Part model, mm, in its own coordinate system. Face numbers are marked on the shaded views. A direction names the side the tool comes from. Coordinates: 2 decimals unless noted, no trailing zeros. Order: outer loops, then holes, each group sorted by start corner. A loop starts at its lowest first (then second) coordinate and runs counter-clockwise, first axis right, second up.
from build123d import *

# Parameters (mm, degrees)
SKETCH1_W           = 580
SKETCH1_H           = 410
BOSS_EXTRUDE1_DEPTH = 140
SKETCH3_W           = 550
SKETCH3_H           = 380
CUT_EXTRUDE1_DEPTH  = 10
SKETCH2_W           = 225
SKETCH2_H           = 350
CUT_EXTRUDE2_DEPTH  = 40
CUT_EXTRUDE3_DEPTH  = 80
FILLET1_R           = 35
SKETCH6_W           = 70
SKETCH6_H           = 70
BOSS_EXTRUDE2_DEPTH = 280
FILLET2_R           = 20


with BuildPart() as part:
    # Sketch1 → Boss-Extrude1 (new body)
    with BuildSketch(Plane(origin=(0, 0, 0), x_dir=(1, 0, 0), z_dir=(0, 1, 0))):
        with Locations((290, 205)):
            Rectangle(SKETCH1_W, SKETCH1_H)
    extrude(amount=-BOSS_EXTRUDE1_DEPTH)

    # Sketch3 → Cut-Extrude1 (cut)
    with BuildSketch(Plane(origin=(0, 0, 0), x_dir=(1, 0, 0), z_dir=(0, 1, 0))):
        with Locations((290, 205)):
            Rectangle(SKETCH3_W, SKETCH3_H)
    extrude(amount=-CUT_EXTRUDE1_DEPTH, mode=Mode.SUBTRACT)

    # Sketch2 → Cut-Extrude2 (cut)
    with BuildSketch(Plane(origin=(0, -10, 0), x_dir=(1, 0, 0), z_dir=(0, 1, 0))):
        with Locations((142.5, 205)):
            Rectangle(SKETCH2_W, SKETCH2_H)
        with Locations((437.5, 205)):
            Rectangle(SKETCH2_W, SKETCH2_H)
    extrude(amount=-CUT_EXTRUDE2_DEPTH, mode=Mode.SUBTRACT)

    # Sketch5 → Cut-Extrude3 (cut)
    with BuildSketch(Plane(origin=(0, -50, 0), x_dir=(1, 0, 0), z_dir=(0, 1, 0))):
        Polygon((30, 320), (90, 380), (255, 380), (255, 30), (90, 30), (30, 90), align=None)
        Polygon((550, 90), (490, 30), (325, 30), (325, 380), (490, 380), (550, 320), align=None)
    extrude(amount=-CUT_EXTRUDE3_DEPTH, mode=Mode.SUBTRACT)

    # Fillet1
    fillet1_edges = [part.edges().sort_by_distance(p)[0] for p in [
        (15, -5, -15),
        (15, -5, -395),
        (565, -5, -395),
        (565, -5, -15),
        (0, -70, -410),
        (580, -70, -410),
        (580, -70, 0),
        (0, -70, 0),
    ]]
    fillet(fillet1_edges, radius=FILLET1_R)

    # Sketch6 → Boss-Extrude2 (add)
    with BuildSketch(Plane.XZ.offset(140)):
        with Locations((65, -65)):
            Rectangle(SKETCH6_W, SKETCH6_H)
        with Locations((515, -65)):
            Rectangle(SKETCH6_W, SKETCH6_H)
        with Locations((515, -345)):
            Rectangle(SKETCH6_W, SKETCH6_H)
        with Locations((65, -345)):
            Rectangle(SKETCH6_W, SKETCH6_H)
    extrude(amount=BOSS_EXTRUDE2_DEPTH)

    # Fillet2
    fillet2_edges = [part.edges().sort_by_distance(p)[0] for p in [
        (30, -30, -30),
        (30, -30, -380),
        (255, -70, -380),
        (255, -70, -30),
        (550, -30, -380),
        (550, -30, -30),
        (325, -70, -30),
        (325, -70, -380),
    ]]
    fillet(fillet2_edges, radius=FILLET2_R)


solid = part.part
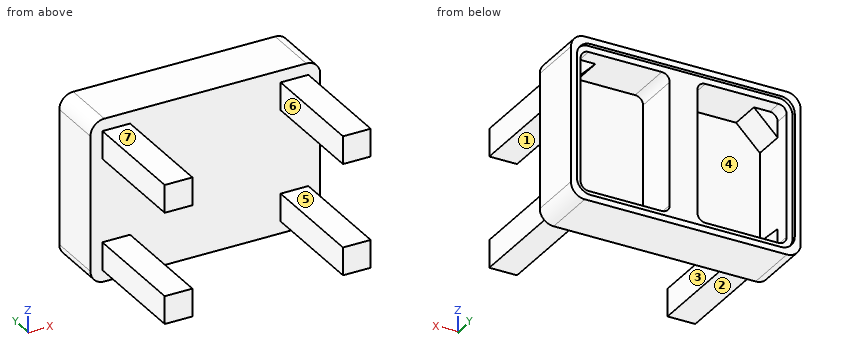
Q1. Mould opens along Z. For the marked faces 1, 2, 3 and 4 say: pulls with the +Z half, pulls with the -Z half, needs draft (parallel to the pull), parting line crosses it, or undercut.
Results list:
face 1: undercut
face 2: pulls with the -Z half
face 3: needs draft
face 4: undercut
Q2. Cut at A-A on y = -334.5. Write the cut outline in (x, z).
Results list:
outline: (30, -380) - (100, -380) - (100, -310) - (30, -310) - close; (30, -100) - (100, -100) - (100, -30) - (30, -30) - close; (480, -380) - (550, -380) - (550, -310) - (480, -310) - close; (480, -100) - (550, -100) - (550, -30) - (480, -30) - close
Q3. Cut at C-C on z = -271. Write the cut outline in (x, y).
Results list:
outline: (0, -140) - (580, -140) - (580, 0) - (565, 0) - (565, -10) - (550, -10) - (550, -130) - (325, -130) - (325, -10) - (255, -10) - (255, -130) - (30, -130) - (30, -10) - (15, -10) - (15, 0) - (0, 0) - close
Q4. Which spindle directions (+Z, -Z, +X, -X, +Y, -Y) get a long thin tool onto all of the face, cutting with end or side? Do the marked faces 5, 6 and 7. Say none if no direction does.
Results list:
face 5: +X, -X, -Y
face 6: +Z, -Z, -Y
face 7: +Z, +X, -X, -Y
Q5. Cut at B-B on y = -31. Write the cut outline in (x, z), and give its area (3 significant figures).
Results list:
outline: (0, -375) arc R35 ccw to (35, -410) - (545, -410) arc R35 ccw to (580, -375) - (580, -35) arc R35 ccw to (545, 0) - (35, 0) arc R35 ccw to (0, -35) - close; hole (30, -360) arc R20 ccw to (50, -380) - (235, -380) arc R20 ccw to (255, -360) - (255, -50) arc R20 ccw to (235, -30) - (50, -30) arc R20 ccw to (30, -50) - close; hole (325, -360) arc R20 ccw to (345, -380) - (530, -380) arc R20 ccw to (550, -360) - (550, -50) arc R20 ccw to (530, -30) - (345, -30) arc R20 ccw to (325, -50) - close
area: 79,900 mm2
Q6. Pin check, flat tips, straight feed: pin 1 Ø21 at (x, y) = (69, -257) entering from +Z; pin 2 Ø21 at (x, y) = (52, -303) entering from -Z; pin 3 Ø18 at (x, z) = (530.5, -359) entering from +Y. Stop position of each tip, or through.
Results list:
pin 1: stops at z = -30
pin 2: stops at z = -380
pin 3: stops at y = -50
Q7. Wall check: line 1 along X through (y, z) = (-47, -177); line 2 along Z through (x, y) = (84, -220); line 3 along Z through (x, y) = (232, -62.5). Give the ranges that are in metal, low to high.
Results list:
line 1: x = 0 to 30, 255 to 325, 550 to 580
line 2: z = -380 to -310, -100 to -30
line 3: z = -410 to -380, -30 to 0
Q8. Cut at D-D on x = 374.5. Write the cut outline in (y, z), and give its area (3 significant figures).
Results list:
outline: (-140, -410) - (0, -410) - (0, -395) - (-10, -395) - (-10, -380) - (-130, -380) - (-130, -30) - (-10, -30) - (-10, -15) - (0, -15) - (0, 0) - (-140, 0) - close
area: 11,600 mm2
